Here's how the part is built. I have some questions about the finished solid (model axes, mm). A direction names the side the tool comes from. Round coordinates to 2 decimals unless told otherwise and drop trailing zeros. Write each loop counter-clockwise with the first axis right and the second up, starting at its lowest first coordinate (ties: lowest second). Pieces come first, ordered by that corner, then holes. Notation, with made-up numbers: (59, 85.25) -> (104, 85.25) arc R17 cw to (104, 115.25) -> close; hole circle Ø11 at (52.5, 11). An arc over 180 degrees is marked (long way). Answer as CSV lines item,"result".
```python
from build123d import *
from OCP.BRepFilletAPI import BRepFilletAPI_MakeFillet

# Parameters (mm, degrees)
SKETCH1_W           = 6.5
SKETCH1_H           = 6.5
BOSS_EXTRUDE1_DEPTH = 4
SKETCH5_W           = 6.5
SKETCH5_H           = 6.5
BOSS_EXTRUDE2_DEPTH = 8
SKETCH2_W           = 4.5
SKETCH2_H           = 4.5
CUT_EXTRUDE1_DEPTH  = 4
SKETCH10_W          = 1.75
SKETCH10_H          = 1.5
CUT_EXTRUDE3_DEPTH  = 11.024968828
FILLET7_R1          = 0.5
FILLET7_R2          = 1.5
BOSS_EXTRUDE3_DEPTH = 2
SKETCH12_W          = 1
SKETCH12_H          = 4.5
CUT_EXTRUDE4_DEPTH  = 5.5
SKETCH14_W          = 1
SKETCH14_H          = 4.5
CUT_EXTRUDE5_DEPTH  = 5.5
SKETCH15_W          = 4.5
SKETCH15_H          = 1
CUT_EXTRUDE6_DEPTH  = 5.5


with BuildPart() as part:
    # Sketch1 → Boss-Extrude1 (new, symmetric)
    with BuildSketch(Plane.XY):
        with Locations((3.25, 3.25)):
            Rectangle(SKETCH1_W, SKETCH1_H)
        with Locations((-3.25, 3.25)):
            Rectangle(SKETCH1_W, SKETCH1_H)
    extrude(amount=BOSS_EXTRUDE1_DEPTH, both=True)

    # Sketch5 → Boss-Extrude2 (add)
    with BuildSketch(Plane.XY.offset(4)):
        with Locations((0, -3.25)):
            Rectangle(SKETCH5_W, SKETCH5_H)
    extrude(amount=-BOSS_EXTRUDE2_DEPTH)

    # Sketch2 → Cut-Extrude1 (cut)
    with BuildSketch(Plane.XY.offset(4)):
        with Locations((3.25, 3.25)):
            Rectangle(SKETCH2_W, SKETCH2_H)
        with Locations((-3.25, 3.25)):
            Rectangle(SKETCH2_W, SKETCH2_H)
        with Locations((0, -3.25)):
            Rectangle(SKETCH2_W, SKETCH2_H)
    extrude(amount=-CUT_EXTRUDE1_DEPTH, mode=Mode.SUBTRACT)

    # Sketch10 → Cut-Extrude3 (cut, through all)
    with BuildSketch(Plane.XY):
        with Locations((1.875, 3.25)):
            Rectangle(SKETCH10_W, SKETCH10_H)
        with Locations((-4.625, 3.25)):
            Rectangle(SKETCH10_W, SKETCH10_H)
        with Locations((4.625, 3.25)):
            Rectangle(SKETCH10_W, SKETCH10_H)
        with Locations((-1.875, 3.25)):
            Rectangle(SKETCH10_W, SKETCH10_H)
        with Locations((-1.375, -3.25)):
            Rectangle(SKETCH10_W, SKETCH10_H)
        with Locations((1.375, -3.25)):
            Rectangle(SKETCH10_W, SKETCH10_H)
    extrude(amount=-CUT_EXTRUDE3_DEPTH, mode=Mode.SUBTRACT)

    # Fillet7: one fillet with a radius per group of edges: ONE call of the kernel's fillet builder (fillet() takes one radius for all edges)
    fillet7_edges_1 = [part.edges().sort_by_distance(p)[0] for p in [
        (-6.5, 0, 0),
        (-6.5, 6.5, 0),
        (6.5, 6.5, 0),
        (6.5, 0, 0),
        (-3.25, -6.5, 0),
        (3.25, -6.5, 0),
    ]]
    fillet7_edges_2 = [part.edges().sort_by_distance(p)[0] for p in [
        (-3.25, 0, 0),
        (3.25, 0, 0),
    ]]
    fillet7 = BRepFilletAPI_MakeFillet(part.part.solid().wrapped)
    for e in fillet7_edges_1:
        fillet7.Add(FILLET7_R1, e.wrapped)
    for e in fillet7_edges_2:
        fillet7.Add(FILLET7_R2, e.wrapped)
    add(Compound.cast(fillet7.Shape()), mode=Mode.REPLACE)

    # Sketch11 → Boss-Extrude3 (add)
    with BuildSketch(Plane.XY.offset(-4)):
        with BuildLine():
            ThreePointArc((-6.662391677, -12.878763029), (1.7135e-05, -14.5), (6.662422116, -12.878747282))
            ThreePointArc((6.662422116, -12.878747282), (6.529952292, -10.609320257), (4.978591095, -8.947656719))
            ThreePointArc((4.978591095, -8.947656719), (4.08034863, -4.787651774), (8.335817539, -4.728787212))
            ThreePointArc((8.335817539, -4.728787212), (11.36788446, -5.887108435), (13.95725976, -3.93))
            ThreePointArc((13.95725976, -3.93), (12.614166243, 7.150720942), (3.796390173, 13.994192426))
            ThreePointArc((3.796390173, 13.994192426), (2.811770094, 12.543018162), (2.695822199, 10.793178304))
            ThreePointArc((2.695822199, 10.793178304), (0, 7.5), (-2.695822199, 10.793178304))
            ThreePointArc((-2.695822199, 10.793178304), (-2.811770094, 12.543018162), (-3.796390173, 13.994192426))
            ThreePointArc((-3.796390173, 13.994192426), (-12.614205329, 7.150651992), (-13.957216796, -3.930152581))
            ThreePointArc((-13.957216796, -3.930152581), (-11.367821604, -5.887138898), (-8.335824842, -4.728795885))
            ThreePointArc((-8.335824842, -4.728795885), (-4.08035569, -4.787642902), (-4.978581003, -8.947651551))
            ThreePointArc((-4.978581003, -8.947651551), (-6.529938219, -10.609328183), (-6.662391677, -12.878763029))
        make_face()
        with BuildLine():
            Line((-3.25, -1.5), (-3.25, -6))
            ThreePointArc((-3.25, -6), (-3.103553391, -6.353553391), (-2.75, -6.5))
            Line((-2.75, -6.5), (2.75, -6.5))
            ThreePointArc((2.75, -6.5), (3.103553391, -6.353553391), (3.25, -6))
            Line((3.25, -6), (3.25, -1.5))
            ThreePointArc((3.25, -1.5), (3.689339828, -0.439339828), (4.75, 0))
            Line((4.75, 0), (6, 0))
            ThreePointArc((6, 0), (6.353553391, 0.146446609), (6.5, 0.5))
            Line((6.5, 0.5), (6.5, 6))
            ThreePointArc((6.5, 6), (6.353553391, 6.353553391), (6, 6.5))
            Line((6, 6.5), (-6, 6.5))
            ThreePointArc((-6, 6.5), (-6.353553391, 6.353553391), (-6.5, 6))
            Line((-6.5, 6), (-6.5, 0.5))
            ThreePointArc((-6.5, 0.5), (-6.353553391, 0.146446609), (-6, 0))
            Line((-6, 0), (-4.75, 0))
            ThreePointArc((-4.75, 0), (-3.689339828, -0.439339828), (-3.25, -1.5))
        make_face(mode=Mode.SUBTRACT)
    extrude(amount=BOSS_EXTRUDE3_DEPTH)

    # Sketch12 → Cut-Extrude4 (cut)
    with BuildSketch(Plane.ZY.offset(6.5)):
        with Locations((2.5, 3.25)):
            Rectangle(SKETCH12_W, SKETCH12_H)
    extrude(amount=-CUT_EXTRUDE4_DEPTH, mode=Mode.SUBTRACT)

    # Sketch14 → Cut-Extrude5 (cut)
    with BuildSketch(Plane(origin=(6.5, 0, 0), x_dir=(0, 0, -1), z_dir=(1, 0, 0))):
        with Locations((-2.5, 3.25)):
            Rectangle(SKETCH14_W, SKETCH14_H)
    extrude(amount=-CUT_EXTRUDE5_DEPTH, mode=Mode.SUBTRACT)

    # Sketch15 → Cut-Extrude6 (cut)
    with BuildSketch(Plane.XZ.offset(6.5)):
        with Locations((0, 2.5)):
            Rectangle(SKETCH15_W, SKETCH15_H)
    extrude(amount=-CUT_EXTRUDE6_DEPTH, mode=Mode.SUBTRACT)


solid = part.part
```
1. Suppose I cut it at B-B on z = 1.5. Please give me the cut outline in (x, y), and give its area (3 significant figures).
Numbers:
outline,"(-6.5, 0.5) arc R0.5 ccw to (-6, 0) -> (-4.75, 0) arc R1.5 cw to (-3.25, -1.5) -> (-3.25, -6) arc R0.5 ccw to (-2.75, -6.5) -> (2.75, -6.5) arc R0.5 ccw to (3.25, -6) -> (3.25, -1.5) arc R1.5 cw to (4.75, 0) -> (6, 0) arc R0.5 ccw to (6.5, 0.5) -> (6.5, 6) arc R0.5 ccw to (6, 6.5) -> (-6, 6.5) arc R0.5 ccw to (-6.5, 6) -> close; hole (-5.5, 1) -> (-1, 1) -> (-1, 5.5) -> (-5.5, 5.5) -> close; hole (-2.25, -5.5) -> (2.25, -5.5) -> (2.25, -1) -> (-2.25, -1) -> close; hole (1, 1) -> (5.5, 1) -> (5.5, 5.5) -> (1, 5.5) -> close"
area,"66.6 mm^2"
2. Suppose I cut it at D-D on z = -2.5. Count the separate pieces of the cut face and the enclosed holes in it, and give its area (3 significant figures).
Numbers:
separate pieces,"1"
enclosed holes,"6"
area,"513 mm^2"
3. For pin 1 Ø1.9 at (x, z) = (-1.5, -2.5) entering from +Y; pin 2 Ø1.3 at (x, y) = (1, -3) entering from +Z; pin 3 Ø8 at (x, y) = (-3, -6.5) entering from +Z; pin 4 Ø2 at (x, z) = (4.5, 1) entering from -Y, each with a flat end and sliding along its axis, tell me the tip position at first contact or that it passes through.
Numbers:
pin 1,"stops at y = 9"
pin 2,"stops at z = 0"
pin 3,"stops at z = 4"
pin 4,"stops at y = -0.67"
4. If we mould it in two halves opening along X, with no side actions, what happens to faces 1 (the face through (5, 0, 1)), 2 (the face through (-6.5, 3, 1)), 3 (the face through (5.5, 3, 0))? For each: released by +X, released by -X, zero draft, split by the parting line, or undercut.
Numbers:
face 1,"zero draft"
face 2,"released by -X"
face 3,"undercut"
5. Suppose I cut it at C-C on y = 10.25. Please give me the cut outline in (x, z).
Numbers:
outline,"(-10.26, -4) -> (-2.75, -4) -> (-2.75, -2) -> (-10.26, -2) -> close; (2.75, -4) -> (10.26, -4) -> (10.26, -2) -> (2.75, -2) -> close"
6. Suppose I cut it at A-A on x = 0. Please give me the cut outline in (y, z).
Numbers:
outline,"(-14.5, -4) -> (7.5, -4) -> (7.5, -2) -> (6.5, -2) -> (6.5, 4) -> (-1, 4) -> (-1, 0) -> (-5.5, 0) -> (-5.5, 2) -> (-6.5, 2) -> (-6.5, -2) -> (-14.5, -2) -> close; (-6.5, 3) -> (-5.5, 3) -> (-5.5, 4) -> (-6.5, 4) -> close"
7. On a 3-axis mill with a long thin cutter (end or side, diameter ignored), from which of +Z, -Z, +X, -X, +Y, -Y can I reach the whole of each face in a straight line? I mean faces 4 (the face through (6.5, 3, 1)), 5 (the face through (-1, 3, 1)), 6 (the face through (0, 6.5, 1)), 7 (the face through (-1, -2.5, -2)). Say none if no direction works.
Numbers:
face 4,"+Z, +X, +Y, -Y"
face 5,"+Z"
face 6,"+Z, +X, -X, +Y"
face 7,"+Z, -Z"
8. If I drill on line 1 (Y direction, x = -1.5, z = 1.25); line 2 (Y direction, x = 1.75, z = -0.75); line 3 (Y direction, x = -0.5, z = 0.75), over which ranges is the centre line in solid material (lowest first)?
Numbers:
line 1,"y = -6.5 to -5.5, -1 to 1, 5.5 to 6.5"
line 2,"y = -6.5 to -4, -2.5 to 2.5, 4 to 6.5"
line 3,"y = -6.5 to -5.5, -1 to 6.5"
